from build123d import *

# Parameters (mm, degrees)
BOSS_EXTRUDE1_DEPTH     = 38
FILLET1_R               = 4
FILLET2_R               = 8
CUT_EXTRUDE1_DEPTH      = 1
CUT_EXTRUDE1_DEPTH_BACK = 13
FILLET3_R               = 4
SKETCH4_R               = 8
CUT_EXTRUDE4_DEPTH      = 82.000266539
CUT_EXTRUDE5_DEPTH      = 51.051633202
CUT_EXTRUDE5_DEPTH_BACK = 45.963614062


with BuildPart() as part:
    # Sketch1 → Boss-Extrude1 (new body, symmetric)
    with BuildSketch(Plane.YZ):
        with BuildLine():
            Line((9.12257761, 0), (70, 0))
            Line((70, 0), (70, 3))
            Line((70, 3), (9.12257761, 3))
            ThreePointArc((9.12257761, 3), (5.949164249, 4.564954284), (5.258874305, 8.03527618))
            Line((5.258874305, 8.03527618), (23.211541616, 75.035542719))
            ThreePointArc((23.211541616, 75.035542719), (27.110151064, 78.000114231), (30.956427827, 74.967954121))
            Line((30.956427827, 74.967954121), (39.477634655, 40.791260242))
            ThreePointArc((39.477634655, 40.791260242), (41.753922912, 37.715033217), (45.538722765, 37.149391089))
            Line((45.538722765, 37.149391089), (58.152567206, 40.294375732))
            ThreePointArc((58.152567206, 40.294375732), (61.228794232, 42.570663989), (61.79443636, 46.355463841))
            Line((61.79443636, 46.355463841), (60.826748777, 50.236646746))
            Line((60.826748777, 50.236646746), (57.915861598, 49.510881059))
            Line((57.915861598, 49.510881059), (58.883549181, 45.629698154))
            ThreePointArc((58.883549181, 45.629698154), (58.65729233, 44.115778213), (57.426801519, 43.205262911))
            Line((57.426801519, 43.205262911), (44.812957078, 40.060278268))
            ThreePointArc((44.812957078, 40.060278268), (43.299037137, 40.286535119), (42.388521834, 41.517025929))
            Line((42.388521834, 41.517025929), (33.867315005, 75.693719808))
            ThreePointArc((33.867315005, 75.693719808), (27.13633067, 81), (20.313764138, 75.811999854))
            Line((20.313764138, 75.811999854), (2.361096826, 8.811733316))
            ThreePointArc((2.361096826, 8.811733316), (3.569104228, 2.738669997), (9.12257761, 0))
        make_face()
    extrude(amount=BOSS_EXTRUDE1_DEPTH, both=True)

    # Fillet1
    fillet1_edges = [part.edges().sort_by_distance(p)[0] for p in [
        (-38, 59.371305188, 49.873763903),
        (38, 59.371305188, 49.873763903),
    ]]
    fillet(fillet1_edges, radius=FILLET1_R)

    # Fillet2
    fillet2_edges = [part.edges().sort_by_distance(p)[0] for p in [
        (-38, 70, 1.5),
        (38, 70, 1.5),
    ]]
    fillet(fillet2_edges, radius=FILLET2_R)

    # Sketch2 → Cut-Extrude1 (cut, two sides)
    with BuildSketch(Plane(origin=(0, 0, 0), x_dir=(1, 0, 0), z_dir=(0, 0, -1))) as cut_extrude1_sk:
        Polygon((-25, -70), (-6.612779769, -38), (4.912194323, -38), (25, -70), align=None)
    extrude(amount=CUT_EXTRUDE1_DEPTH, mode=Mode.SUBTRACT)
    extrude(cut_extrude1_sk.sketch, amount=-CUT_EXTRUDE1_DEPTH_BACK, mode=Mode.SUBTRACT)

    # Fillet3
    fillet3_edges = [part.edges().sort_by_distance(p)[0] for p in [
        (4.912194323, 38, 1.5),
        (-6.612779769, 38, 1.5),
    ]]
    fillet(fillet3_edges, radius=FILLET3_R)

    # Sketch4 → Cut-Extrude4 (cut, through all)
    with BuildSketch(Plane(origin=(0, 0, 0), x_dir=(1, 0, 0), z_dir=(0, 0, -1))):
        with Locations((0, -2.12257761)):
            Circle(SKETCH4_R)
    extrude(amount=-CUT_EXTRUDE4_DEPTH, mode=Mode.SUBTRACT)

    # Sketch6 → Cut-Extrude5 (cut, two sides)
    with BuildSketch(Plane(origin=(0, -6.780848473, 27.196497771), x_dir=(1, 0, 0), z_dir=(0, -0.241921896, 0.970295726))) as cut_extrude5_sk:
        Polygon((-19, 71.173279191), (-7.452994616, 51.173279191), (7.452994616, 51.173279191), (19, 71.173279191), align=None)
    extrude(amount=CUT_EXTRUDE5_DEPTH, mode=Mode.SUBTRACT)
    extrude(cut_extrude5_sk.sketch, amount=-CUT_EXTRUDE5_DEPTH_BACK, mode=Mode.SUBTRACT)


solid = part.part
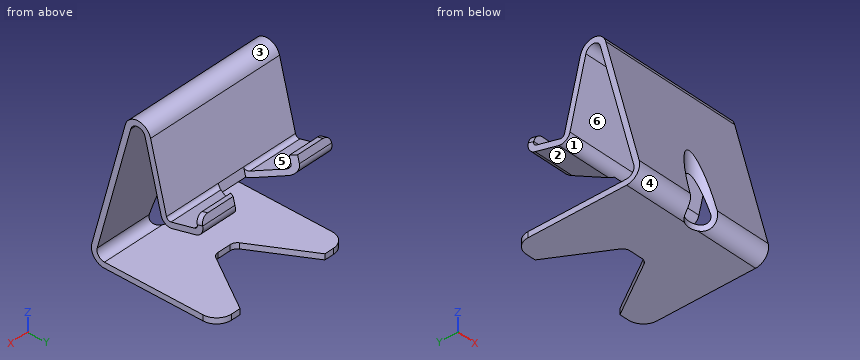
Could you check a few things on this model? Use its own coordinates, in mm. Face numbers are marked on the shaded views. A direction names the side the tool comes from. Round coordinates to 2 decimals unless told otherwise and drop trailing zeros. Order: outer loops, then holes, each group sorted by start corner. A loop starts at its lowest first (then second) coordinate and runs counter-clockwise, first axis right, second up.
Q1. Which directions (+Z, -Z, +X, -X, +Y, -Y) give clear straight access to the entire face, cutting with the end or side of a thin tool? Please do the marked faces 1, 2 and 3.
Geometry says:
face 1: +X, -X
face 2: +X, -X, +Y
face 3: +Z, +X, -X
Q2. Imagine slicing it at C-C, the plane z = 53. List the corners of the cut face in (x, y) for me, then the cut area to 3 significant figures.
Geometry says:
outline: (-38, 14.2) - (38, 14.2) - (38, 17.31) - (-38, 17.31) - close; (-38, 36.43) - (38, 36.43) - (38, 39.53) - (-38, 39.53) - close
area: 471 mm2
Q3. Imagine slicing it at D-D, the plane x = 0. List the corners of the cut face in (y, z) for me.
Geometry says:
outline: (10.12, 0) - (38, 0) - (38, 3) - (10.12, 3) - close; (10.12, 26.19) - (23.21, 75.04) arc R4 cw to (30.96, 74.97) - (39.48, 40.79) arc R5 ccw to (43.5, 37.07) - (33.87, 75.69) arc R7 ccw to (20.31, 75.81) - (10.12, 37.78) - close
Q4. Imagine slicing it at A-A, the plane y = 55.5. List the corners of the cut face in (x, z) for me, then the cut area to 3 significant figures.
Geometry says:
outline: (-38, 0) - (-16.67, 0) - (-16.67, 3) - (-38, 3) - close; (-38, 39.63) - (-14.53, 39.63) - (-14.97, 42.72) - (-38, 42.72) - close; (14.53, 39.63) - (38, 39.63) - (38, 42.72) - (14.97, 42.72) - close; (15.9, 0) - (38, 0) - (38, 3) - (15.9, 3) - close
area: 274 mm2
Q5. Imagine slicing it at B-B, the plane x = 26.5. List the corners of the cut face in (y, z) for me, then the cut area to 3 significant figures.
Geometry says:
outline: (2.36, 8.81) arc R7 ccw to (9.12, 0) - (70, 0) - (70, 3) - (9.12, 3) arc R4 cw to (5.26, 8.04) - (23.21, 75.04) arc R4 cw to (30.96, 74.97) - (39.48, 40.79) arc R5 ccw to (45.54, 37.15) - (58.15, 40.29) arc R5 ccw to (61.79, 46.36) - (60.83, 50.24) - (57.92, 49.51) - (58.88, 45.63) arc R2 cw to (57.43, 43.21) - (44.81, 40.06) arc R2 cw to (42.39, 41.52) - (33.87, 75.69) arc R7 ccw to (20.31, 75.81) - close
area: 654 mm2
Q6. I'm going to push flat-ended pins straight in: P1, Ø1.5, axis at x = -20, y = 50.5, coming from the -Z side; P2, Ø1.5, axis at x = 13, z = 24.5, coming from the +Y side; P3, Ø5, axis at x = -15, z = 28, coming from the -Y side; P4, Ø8, axis at x = -9, z = 12, coming from the -Y side. Where does each tip first touch, or does it pass through?
Geometry says:
P1: stops at z = 0
P2: stops at y = 9.87
P3: stops at y = 6.83
P4: stops at y = 2.19
Q7. Thinking about a two-plate mould opening in Z: for the marked faces 4, 5 and 6, which applies, released by +Z, released by -Z, zero draft, split by the parting line, or undercut?
Geometry says:
face 4: split by the parting line
face 5: released by +Z
face 6: undercut
Q8. Please list where these lines run through material, in increasing order: probe 1 along Z at (x, y) = (-20.5, 44); probe 2 along Y at (x, z) = (33, 52); probe 3 along Y at (x, z) = (29, 66).
Geometry says:
probe 1: z = 0 to 3, 37.01 to 40.03
probe 2: y = 13.93 to 17.04, 36.68 to 39.77
probe 3: y = 17.68 to 20.79, 33.19 to 36.28
